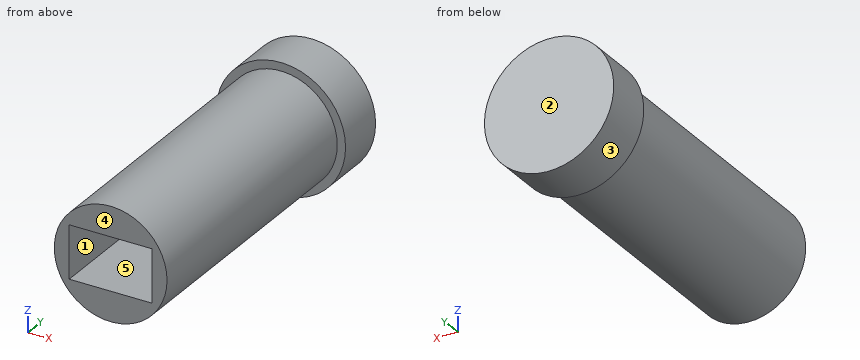
```python
from build123d import *

# Parameters (mm, degrees)
SKETCH_4_W          = 25
SKETCH_4_H          = 16
CUT_EXTRUDE_1_DEPTH = 65


with BuildPart() as part:
    # Эскиз3 → Повернуть2 (revolve)
    with BuildSketch(Plane.XY):
        Polygon((0, 0), (17, 0), (17, 85), (19.5, 85), (19.5, 100), (0, 100), align=None)
    revolve(axis=Axis((0, 0, 0), (0, 1, 0)))

    # Эскиз4 → Вырез-Вытянуть1 (cut)
    with BuildSketch(Plane.XZ):
        Rectangle(SKETCH_4_W, SKETCH_4_H)
    extrude(amount=-CUT_EXTRUDE_1_DEPTH, mode=Mode.SUBTRACT)


solid = part.part
```
Could you check a few things on this model? Use its own coordinates, in mm. Face numbers are marked on the shaded views. A direction names the side the tool comes from. Give positions to 0.01 mm unless a question says otherwise; leave off trailing zeros. Order: outer loops, then holes, each group sorted by start corner. A loop starts at its lowest first (then second) coordinate and runs counter-clockwise, first axis right, second up.
Q1. We'd pull the mould along Z, two halves only. Please class the marked faces 1, 2 and 3: +Z half, -Z half, draft (parallel to the pull), parting line (faces both ways), or undercut.
Q2. Suppose I cut it at C-C, the plane z = 6.5. Write out the boundary of the cut face in (x, y).
Q3. For the marked faces 4 and 5, which set-ups out of +Z, -Z, +X, -X, +Y, -Y let a thin tool reach every point of the face, with its end or its side?
Q4. If I drill on line 1 along Z through (x, y) = (0.5, 28.5); line 2 along Y through (x, z) = (-6, 5); line 3 along X through (y, z) = (35.5, 11.5), over which ranges is the centre line in solid material (lowest first)?
Q5. I'm going to push flat-ended pins straight in: P1, Ø12.5, axis at x = 3.5, y = 29.5, coming from the +Z side; P2, Ø4, axis at x = 13.5, y = 17, coming from the -Z side; P3, Ø8, axis at y = 47, z = -1.5, coming from the +X side; P4, Ø1, axis at x = -8, z = -9.5, coming from the -Y side. Where does each tip first touch, or does it pass through?
Q6. Suppose I cut it at D-D, the plane y = 67.5. Write out the boundary of the cut face in (x, z), and give its area (3 significant figures).
Q7. Suppose I cut it at A-A, the plane x = 0. Write out the boundary of the cut face in (y, z), and give its area (4 significant figures).
Q8. Suppose I cut it at B-B, the plane y = 12. Write out the boundary of the cut face in (x, z).
Solution:
1. face 1: undercut
1. face 2: draft
1. face 3: parting line
2. outline: (-18.38, 85) - (-15.71, 85) - (-15.71, 0) - (-12.5, 0) - (-12.5, 65) - (12.5, 65) - (12.5, 0) - (15.71, 0) - (15.71, 85) - (18.38, 85) - (18.38, 100) - (-18.38, 100) - close
3. face 4: +Z, -Z, +X, -X, -Y
3. face 5: -Y
4. line 1: z = -16.99 to -8, 8 to 16.99
4. line 2: y = 65 to 100
4. line 3: x = -12.52 to 12.52
5. P1: stops at z = 17
5. P2: stops at z = -12.52
5. P3: stops at x = 17
5. P4: stops at y = 0
6. outline: circle Ø34 at (0, 0)
6. area: 908 mm2
7. outline: (0, -17) - (85, -17) - (85, -19.5) - (100, -19.5) - (100, 19.5) - (85, 19.5) - (85, 17) - (0, 17) - (0, 8) - (65, 8) - (65, -8) - (0, -8) - close
7. area: 2,435 mm2
8. outline: circle Ø34 at (0, 0); hole (-12.5, -8) - (12.5, -8) - (12.5, 8) - (-12.5, 8) - close
